The listing builds one solid part. Answer for the finished solid, in the listing's coordinates (mm). A direction names the side the tool comes from. Round coordinates to 2 decimals unless told otherwise and drop trailing zeros. Write each loop counter-clockwise with the first axis right and the second up, starting at its lowest first coordinate (ties: lowest second). Pieces come first, ordered by that corner, then holes. Notation, with made-up numbers: (-0.5, 8.5) -> (6.5, 8.5) arc R30 cw to (6.5, 46.5) -> close; hole circle Ø2 at (33, -27.75). An arc over 180 degrees is marked (long way). Write each question's results on one line, items separated by ' | '. Start each with the question number.
```python
from build123d import *

# Parameters (mm, degrees)
CYLINDER002_R     = 1
CYLINDER002_DEPTH = 10
CYLINDER001_R     = 5.5
CYLINDER001_DEPTH = 10
CYLINDER003_R     = 3.5
CYLINDER003_DEPTH = 10
CYLINDER004_R     = 3.5
CYLINDER004_DEPTH = 10
CYLINDER_R        = 5.5
CYLINDER_DEPTH    = 10
CYLINDER005_R     = 4.5
CYLINDER005_DEPTH = 1
CYLINDER006_R     = 4.5
CYLINDER006_DEPTH = 1
BOX_W             = 16
BOX_H             = 9
BOX_DEPTH         = 1


with BuildPart() as cylinder002_post_hole:
    # Cylinder002 → Cylinder002 (new body)
    with BuildSketch(Plane(origin=(9, 6, 0), x_dir=(1, 0, 0), z_dir=(0, 0, 1))):
        Circle(CYLINDER002_R)
    extrude(amount=CYLINDER002_DEPTH)


with BuildPart() as cylinder001_b:
    # Cylinder001 → Cylinder001 (new body)
    with BuildSketch(Plane(origin=(14, 0, 0), x_dir=(1, 0, 0), z_dir=(0, 0, 1))):
        Circle(CYLINDER001_R)
    extrude(amount=CYLINDER001_DEPTH)


with BuildPart() as cylinder003_b2_inner:
    # Cylinder003 → Cylinder003 (new body)
    with BuildSketch(Plane(origin=(17.5, 11.5, 0), x_dir=(1, 0, 0), z_dir=(0, 0, 1))):
        Circle(CYLINDER003_R)
    extrude(amount=CYLINDER003_DEPTH)


with BuildPart() as cylinder004_a2_inner:
    # Cylinder004 → Cylinder004 (new body)
    with BuildSketch(Plane(origin=(4.75, 11.25, 0), x_dir=(1, 0, 0), z_dir=(0, 0, 1))):
        Circle(CYLINDER004_R)
    extrude(amount=CYLINDER004_DEPTH)


with BuildPart() as fusion001:
    # Cylinder → Cylinder (new body)
    with BuildSketch(Plane(origin=(-0.5, 0, 0), x_dir=(1, 0, 0), z_dir=(0, 0, 1))):
        Circle(CYLINDER_R)
    extrude(amount=CYLINDER_DEPTH)

    # Fusion001: union Cylinder002(post_hole), Cylinder001(B), Cylinder003(B2)(inner), Cylinder004(A2)(inner)
    add(cylinder002_post_hole.part)
    add(cylinder001_b.part)
    add(cylinder003_b2_inner.part)
    add(cylinder004_a2_inner.part)


with BuildPart() as cylinder003_b2_outer:
    # Cylinder005 → Cylinder005 (new body)
    with BuildSketch(Plane(origin=(17.5, 11.5, 0), x_dir=(1, 0, 0), z_dir=(0, 0, 1))):
        Circle(CYLINDER005_R)
    extrude(amount=CYLINDER005_DEPTH)


with BuildPart() as cylinder004_a2_outer:
    # Cylinder006 → Cylinder006 (new body)
    with BuildSketch(Plane(origin=(4.75, 11.25, 0), x_dir=(1, 0, 0), z_dir=(0, 0, 1))):
        Circle(CYLINDER006_R)
    extrude(amount=CYLINDER006_DEPTH)


with BuildPart() as cut_button_well:
    # Box → Box (new body)
    with BuildSketch(Plane(origin=(-0.5, 3, 0), x_dir=(1, 0, 0), z_dir=(0, 0, 1))):
        with Locations((8, 4.5)):
            Rectangle(BOX_W, BOX_H)
    extrude(amount=BOX_DEPTH)

    # Fusion: union Cylinder003(B2)(outer), Cylinder004(A2)(outer)
    add(cylinder003_b2_outer.part)
    add(cylinder004_a2_outer.part)

    # Cut: cut Fusion001
    add(fusion001.part, mode=Mode.SUBTRACT)


solid = cut_button_well.part
```
Q1. Determine the mould class of faces 1 (the cylindrical face through (8.87, 6.99, 0.49)), 2 (the flat face through (6.7, 3, 0.5)), 3 (the flat face through (8.1, 9.6, 0)), 4 (the cylindrical face through (4.84, 15.75, 0.49)) for opening direction Y: pulls with the +Y half, pulls with the -Y half, needs draft (parallel to the pull), parting line crosses it, or undercut.
Q2. The part is cut by section B-B, the plane y = 6. Write down the section's boundary in (x, z), then the cut area to 3 significant figures.
Q3. For faces 5 (the flat face through (15.5, 6.4, 0.5)), 6 (the flat face through (11.1, 12, 0.5)), 7 (the flat face through (-0.1, 12, 0.5)), 8 (the cylindrical face through (6.365, 8.145, 0.493)), determine the directions among +Z, -Z, +X, -X, +Y, -Y from which every point of the face is accessible in a straight line to the end or side of a thin tool.
Q4. The part is cut by section A-A, the plane x = 17.5. Write down the section's boundary in (y, z), then the cut area to 3 significant figures.
Q5. The part is cut by section D-D, the plane z = 0.25. Write down the section's boundary in (x, y), then the cut area to 3 significant figures.
Q6. The part is cut by section C-C, the plane y = 11.25. Write down the section's boundary in (x, z).
Q7. Find the intervals of material crossed by line 1 (X direction, y = 11, z = 0.9); line 2 (Y direction, x = 4.75, z = 0.3); line 3 (X direction, y = 14, z = 0.6), in increasing order.
Q8. This flat-tipped pin is pushed along its axis until it touches: pin 1 (5 mm diameter, centred on x = 3, y = 13, fed in from +Z). Where does it stop, or does it pass through?
Answers follow:
1) face 1: undercut | face 2: pulls with the -Y half | face 3: needs draft | face 4: pulls with the +Y half
2) outline: (-0.5, 0) -> (8, 0) -> (8, 1) -> (-0.5, 1) -> close; (10, 0) -> (15.5, 0) -> (15.5, 1) -> (10, 1) -> close | area: 14.0 mm^2
3) face 5: +Z, -Z, -Y | face 6: +Z, -Z, +Y | face 7: +Z, -Z, -X, +Y | face 8: +Z, -Z
4) outline: (7, 0) -> (8, 0) -> (8, 1) -> (7, 1) -> close; (15, 0) -> (16, 0) -> (16, 1) -> (15, 1) -> close | area: 2.00 mm^2
5) outline: (-0.5, 5.5) arc R5.5 cw to (4.11, 3) -> (9.39, 3) arc R5.5 cw to (15.5, 5.29) -> (15.5, 7.47) arc R4.5 ccw (long way) to (13.03, 12) -> (9.19, 12) arc R4.5 ccw to (0.31, 12) -> (-0.5, 12) -> close; hole circle Ø7 at (4.75, 11.25); hole circle Ø2 at (9, 6); hole circle Ø7 at (17.5, 11.5) | area: 124 mm^2
6) outline: (-0.5, 0) -> (1.25, 0) -> (1.25, 1) -> (-0.5, 1) -> close; (8.25, 0) -> (14.01, 0) -> (14.01, 1) -> (8.25, 1) -> close; (20.99, 0) -> (21.99, 0) -> (21.99, 1) -> (20.99, 1) -> close
7) line 1: -0.5 to 1.26, 8.24 to 14.04, 20.96 to 21.97 | line 2: 3 to 7.75, 14.75 to 15.75 | line 3: 1.19 to 2.58, 6.92 to 8.31, 13.76 to 15.05, 19.95 to 21.24
8) pin 1: z = 1
